Drawing for the job (mm, zero at the part's lowest x, y, z). Round coordinates to 2 decimals unless told otherwise and drop trailing zeros. Order: outer loops, then holes, each group sorted by start corner. A loop starts at its lowest first (then second) coordinate and runs counter-clockwise, first axis right, second up. Notation, with made-up numbers: (-18, 58.25) -> (23, 58.25) arc R21 cw to (23, 96.25) -> close; hole circle Ø8 at (49.25, -20). An arc over 180 degrees is marked (long way). Answer as CSV lines item,"result". Start each with the question number.
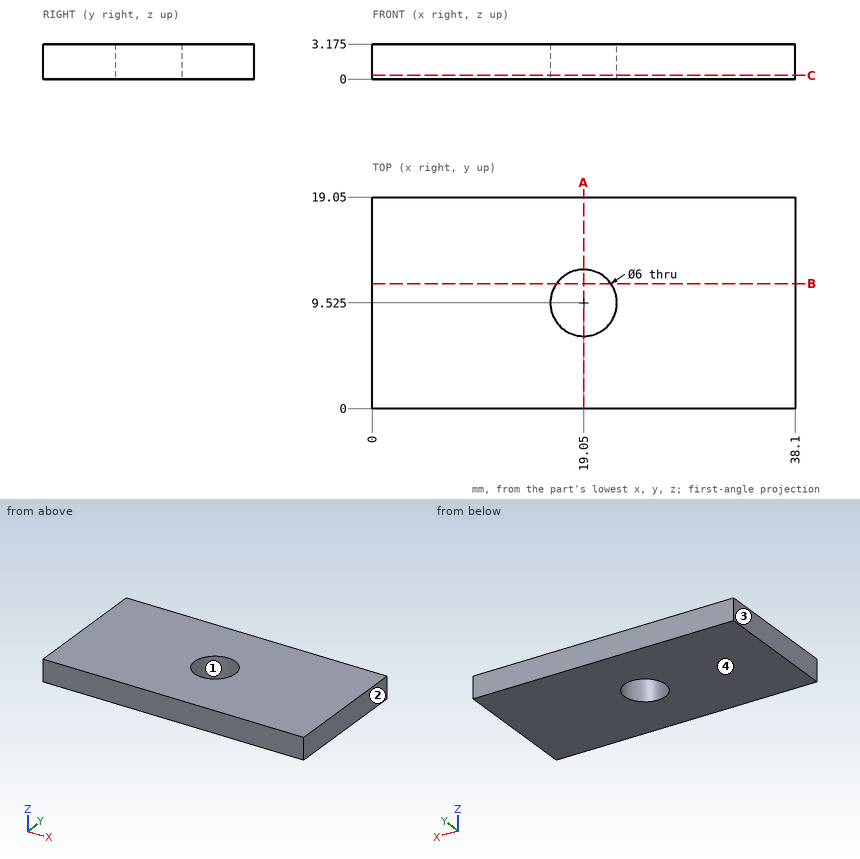
Q1. Slice it at C-C, the plane z = 0.35. Write the cut outline in (x, y) (3 decimals), plus the area to 3 significant figures.
Q2. Slice it at B-B, the plane y = 11.25. Write the cut outline in (x, z) (3 decimals).
Q3. Two-plate mould, pull along X, no slides. Class the marked faces 1, 2, 3 and 4: +X half, -X half, draft (parallel to the pull), parting line (faces both ways), or undercut.
Q4. Slice it at A-A, the plane x = 19.05. Write the cut outline in (y, z) (3 decimals).
Q5. Probe L1, parallel to Y at x = 19.05, z = 1.15 (3 decimals); L2, parallel to X at y = 7, z = 0.4; L3, parallel to X at y = 12.25, z = 2.9. List the from-to ranges inside material, lowest first.
Solutions:
1,outline,"(0, 0) -> (38.1, 0) -> (38.1, 19.05) -> (0, 19.05) -> close; hole circle Ø6 at (19.05, 9.525)"
1,area,"698 mm2"
2,outline,"(0, 0) -> (16.596, 0) -> (16.596, 3.175) -> (0, 3.175) -> close; (21.504, 0) -> (38.1, 0) -> (38.1, 3.175) -> (21.504, 3.175) -> close"
3,face 1,"undercut"
3,face 2,"+X half"
3,face 3,"-X half"
3,face 4,"draft"
4,outline,"(0, 0) -> (6.525, 0) -> (6.525, 3.175) -> (0, 3.175) -> close; (12.525, 0) -> (19.05, 0) -> (19.05, 3.175) -> (12.525, 3.175) -> close"
5,L1,"y = 0 to 6.525, 12.525 to 19.05"
5,L2,"x = 0 to 17.43, 20.67 to 38.1"
5,L3,"x = 0 to 17.8, 20.3 to 38.1"
